Source: three-view drawing plus pictorial views. Frame: mm from the lowest corner of the part. Give positions to 0.01 mm unless a question says otherwise; leave off trailing zeros. Loops run counter-clockwise (first coordinate to the right, second up) from the corner with the lowest first, then second, coordinate; pieces in that order, holes last. Notation, with made-up numbers: (36.5, 75) - (53.5, 75) arc R23 ccw to (53.5, 107) - close; hole circle Ø3 at (-37, -31). An arc over 180 degrees is marked (long way). Answer as a JSON object with one key per item and string values. Group by question number.
(1) Material intervals for L1, parallel to Y at x = 2.54, z = 2.95 (3 decimals); L2, parallel to X at y = 3.35, z = 2.5; L3, parallel to X at y = 1.8, z = 5.5, sorted ascending.
(2) Mould query, pull axis Z, two halves, no side actions, for the marked faces 1, 2, 3 and 4. Classes: +Z half, -Z half, draft (parallel to the pull), parting line (faces both ways), or undercut.
(3) Section query B-B (z = 12.5). Return loops of the section in (x, y), plus the area to 3 significant figures.
(4) Pin query (flat end, axial travel): P1, Ø1.5, axis at x = 2.5, z = 9.5, coming from the -Y side; P2, Ø1, axis at x = 4.5, z = 3, coming from the +Y side; P3, Ø1.5, axis at x = 1.5, z = 11, coming from the -Y side. Return the tip coordinate at first contact, or that it passes through.
(5) Section query A-A (z = 7). Return loops of the section in (x, y), plus the area to 3 significant figures.
(6) Section query C-C (z = 4.5). Return loops of the section in (x, y), plus the area to 3 significant figures.
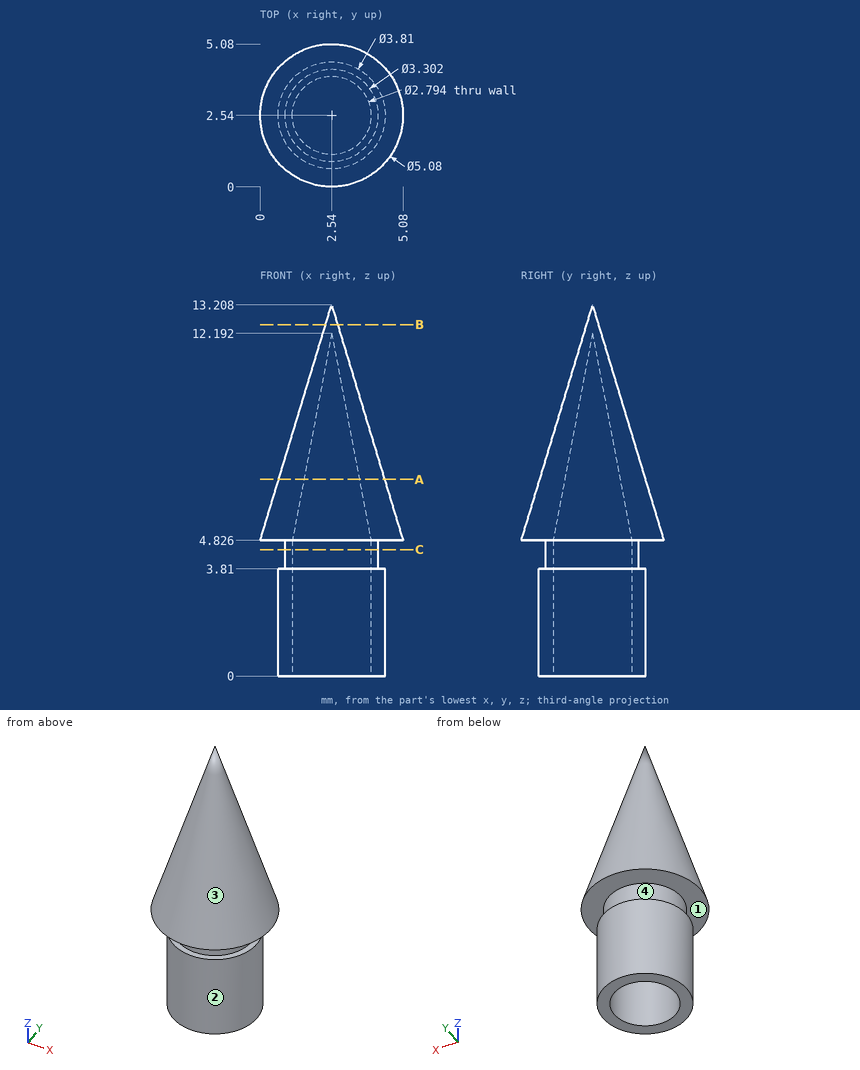
Recorded:
{
 "1": {"L1": "y = 0.635 to 1.143, 3.937 to 4.445", "L2": "x = 0.82 to 1.4, 3.68 to 4.26", "L3": "x = 0.32 to 1.51, 3.57 to 4.76"},
 "2": {"face 1": "undercut", "face 2": "draft", "face 3": "+Z half", "face 4": "undercut"},
 "3": {"outline": "circle Ø0.43 at (2.54, 2.54)", "area": "0.145 mm^2"},
 "4": {"P1": "stops at y = 1.19", "P2": "stops at y = 3.76", "P3": "stops at y = 1.86"},
 "5": {"outline": "circle Ø3.76 at (2.54, 2.54); hole circle Ø1.97 at (2.54, 2.54)", "area": "8.07 mm^2"},
 "6": {"outline": "circle Ø3.3 at (2.54, 2.54); hole circle Ø2.79 at (2.54, 2.54)", "area": "2.43 mm^2"}
}
